from build123d import *

# Parameters (mm, degrees)
SKETCH1_R           = 22.5
BOSS_EXTRUDE1_DEPTH = 200
BOSS_EXTRUDE2_START = 50
BOSS_EXTRUDE2_DEPTH = 100
BOSS_EXTRUDE3_START = -50
SKETCH4_R           = 23.75
SKETCH4_R_2         = 22.25
BOSS_EXTRUDE3_DEPTH = 5
BOSS_EXTRUDE4_START = -171.5
SKETCH4_2_R         = 23.75
SKETCH4_2_R_2       = 22.25
BOSS_EXTRUDE4_DEPTH = 21.5


with BuildPart() as part:
    # Sketch1 → Boss-Extrude1 (new body)
    with BuildSketch(Plane.XY):
        Circle(SKETCH1_R)
        with BuildLine():
            Line((-3.5, 19.691368668), (-3.5, 17.656443583))
            ThreePointArc((-3.5, 17.656443583), (-6.888301783, 16.629831585), (-10.010117255, 14.959864723))
            Line((-10.010117255, 14.959864723), (-11.449026581, 16.39877405))
            ThreePointArc((-11.449026581, 16.39877405), (-14.142135624, 14.142135624), (-16.39877405, 11.449026581))
            Line((-16.39877405, 11.449026581), (-14.959864723, 10.010117255))
            ThreePointArc((-14.959864723, 10.010117255), (-16.629831585, 6.888301783), (-17.656443583, 3.5))
            Line((-17.656443583, 3.5), (-19.691368668, 3.5))
            ThreePointArc((-19.691368668, 3.5), (-20, 0), (-19.691368668, -3.5))
            Line((-19.691368668, -3.5), (-17.656443583, -3.5))
            ThreePointArc((-17.656443583, -3.5), (-16.629831585, -6.888301783), (-14.959864723, -10.010117255))
            Line((-14.959864723, -10.010117255), (-16.39877405, -11.449026581))
            ThreePointArc((-16.39877405, -11.449026581), (-14.142135624, -14.142135624), (-11.449026581, -16.39877405))
            Line((-11.449026581, -16.39877405), (-10.010117255, -14.959864723))
            ThreePointArc((-10.010117255, -14.959864723), (-6.888301783, -16.629831585), (-3.5, -17.656443583))
            Line((-3.5, -17.656443583), (-3.5, -19.691368668))
            ThreePointArc((-3.5, -19.691368668), (0, -20), (3.5, -19.691368668))
            Line((3.5, -19.691368668), (3.5, -17.656443583))
            ThreePointArc((3.5, -17.656443583), (6.888301783, -16.629831585), (10.010117255, -14.959864723))
            Line((10.010117255, -14.959864723), (11.449026581, -16.39877405))
            ThreePointArc((11.449026581, -16.39877405), (14.142135624, -14.142135624), (16.39877405, -11.449026581))
            Line((16.39877405, -11.449026581), (14.959864723, -10.010117255))
            ThreePointArc((14.959864723, -10.010117255), (16.629831585, -6.888301783), (17.656443583, -3.5))
            Line((17.656443583, -3.5), (19.691368668, -3.5))
            ThreePointArc((19.691368668, -3.5), (20, 0), (19.691368668, 3.5))
            Line((19.691368668, 3.5), (17.656443583, 3.5))
            ThreePointArc((17.656443583, 3.5), (16.629831585, 6.888301783), (14.959864723, 10.010117255))
            Line((14.959864723, 10.010117255), (16.39877405, 11.449026581))
            ThreePointArc((16.39877405, 11.449026581), (14.142135624, 14.142135624), (11.449026581, 16.39877405))
            Line((11.449026581, 16.39877405), (10.010117255, 14.959864723))
            ThreePointArc((10.010117255, 14.959864723), (6.888301783, 16.629831585), (3.5, 17.656443583))
            Line((3.5, 17.656443583), (3.5, 19.691368668))
            ThreePointArc((3.5, 19.691368668), (0, 20), (-3.5, 19.691368668))
        make_face(mode=Mode.SUBTRACT)
    extrude(amount=BOSS_EXTRUDE1_DEPTH)

    # Sketch3 → Boss-Extrude2 (add)
    with BuildSketch(Plane.XY.offset(BOSS_EXTRUDE2_START)):
        with BuildLine():
            Line((-2.000027302, 23.665962711), (-0.80077241, 26.237773126))
            ThreePointArc((-0.80077241, 26.237773126), (0, 26.249990002), (0.80077241, 26.237773126))
            Line((0.80077241, 26.237773126), (2.000027302, 23.665962711))
            ThreePointArc((2.000027302, 23.665962711), (2.731879206, 23.592683956), (3.461111111, 23.496778718))
            Line((3.461111111, 23.496778718), (3.461111111, 21.979153985))
            ThreePointArc((3.461111111, 21.979153985), (0, 22.25), (-3.461111111, 21.979153985))
            Line((-3.461111111, 21.979153985), (-3.461111111, 23.496778718))
            ThreePointArc((-3.461111111, 23.496778718), (-2.731879206, 23.592683956), (-2.000027302, 23.665962711))
        make_face()
        with BuildLine():
            Line((17.303950149, 13.98698714), (18.618251721, 14.745799506))
            ThreePointArc((18.618251721, 14.745799506), (19.065924046, 14.162218771), (19.495311261, 13.565055807))
            Line((19.495311261, 13.565055807), (22.322191861, 13.812375813))
            ThreePointArc((22.322191861, 13.812375813), (22.73315819, 13.124995001), (23.122964271, 12.425397313))
            Line((23.122964271, 12.425397313), (21.495338563, 10.100906903))
            ThreePointArc((21.495338563, 10.100906903), (21.797803252, 9.430465185), (22.079362832, 8.750979211))
            Line((22.079362832, 8.750979211), (20.76506126, 7.992166845))
            ThreePointArc((20.76506126, 7.992166845), (19.269065234, 11.125), (17.303950149, 13.98698714))
        make_face()
        with BuildLine():
            Line((20.76506126, -7.992166845), (22.079362832, -8.750979211))
            ThreePointArc((22.079362832, -8.750979211), (21.797803252, -9.430465185), (21.495338563, -10.100906903))
            Line((21.495338563, -10.100906903), (23.122964271, -12.425397313))
            ThreePointArc((23.122964271, -12.425397313), (22.73315819, -13.124995001), (22.322191861, -13.812375813))
            Line((22.322191861, -13.812375813), (19.495311261, -13.565055807))
            ThreePointArc((19.495311261, -13.565055807), (19.065924046, -14.162218771), (18.618251721, -14.745799506))
            Line((18.618251721, -14.745799506), (17.303950149, -13.98698714))
            ThreePointArc((17.303950149, -13.98698714), (19.269065234, -11.125), (20.76506126, -7.992166845))
        make_face()
        with BuildLine():
            Line((3.461111111, -21.979153985), (3.461111111, -23.496778718))
            ThreePointArc((3.461111111, -23.496778718), (2.731879206, -23.592683956), (2.000027302, -23.665962711))
            Line((2.000027302, -23.665962711), (0.80077241, -26.237773126))
            ThreePointArc((0.80077241, -26.237773126), (0, -26.249990002), (-0.80077241, -26.237773126))
            Line((-0.80077241, -26.237773126), (-2.000027302, -23.665962711))
            ThreePointArc((-2.000027302, -23.665962711), (-2.731879206, -23.592683956), (-3.461111111, -23.496778718))
            Line((-3.461111111, -23.496778718), (-3.461111111, -21.979153985))
            ThreePointArc((-3.461111111, -21.979153985), (0, -22.25), (3.461111111, -21.979153985))
        make_face()
        with BuildLine():
            Line((-17.303950149, -13.98698714), (-18.618251721, -14.745799506))
            ThreePointArc((-18.618251721, -14.745799506), (-19.065924046, -14.162218771), (-19.495311261, -13.565055807))
            Line((-19.495311261, -13.565055807), (-22.322191861, -13.812375813))
            ThreePointArc((-22.322191861, -13.812375813), (-22.73315819, -13.124995001), (-23.122964271, -12.425397313))
            Line((-23.122964271, -12.425397313), (-21.495338563, -10.100906903))
            ThreePointArc((-21.495338563, -10.100906903), (-21.797803252, -9.430465185), (-22.079362832, -8.750979211))
            Line((-22.079362832, -8.750979211), (-20.76506126, -7.992166845))
            ThreePointArc((-20.76506126, -7.992166845), (-19.269065234, -11.125), (-17.303950149, -13.98698714))
        make_face()
        with BuildLine():
            Line((-20.76506126, 7.992166845), (-22.079362832, 8.750979211))
            ThreePointArc((-22.079362832, 8.750979211), (-21.797803252, 9.430465185), (-21.495338563, 10.100906903))
            Line((-21.495338563, 10.100906903), (-23.122964271, 12.425397313))
            ThreePointArc((-23.122964271, 12.425397313), (-22.73315819, 13.124995001), (-22.322191861, 13.812375813))
            Line((-22.322191861, 13.812375813), (-19.495311261, 13.565055807))
            ThreePointArc((-19.495311261, 13.565055807), (-19.065924046, 14.162218771), (-18.618251721, 14.745799506))
            Line((-18.618251721, 14.745799506), (-17.303950149, 13.98698714))
            ThreePointArc((-17.303950149, 13.98698714), (-19.269065234, 11.125), (-20.76506126, 7.992166845))
        make_face()
    extrude(amount=BOSS_EXTRUDE2_DEPTH)

    # Sketch4 → Boss-Extrude3 (add)
    with BuildSketch(Plane.XY.offset(200).offset(BOSS_EXTRUDE3_START)):
        with Locations(Location((0, 0, 0), (0, 0, 180))):
            Circle(SKETCH4_R)
        Circle(SKETCH4_R_2, mode=Mode.SUBTRACT)
    extrude(amount=BOSS_EXTRUDE3_DEPTH)

    # Sketch4<2> → Boss-Extrude4 (add)
    with BuildSketch(Plane.XY.offset(200).offset(BOSS_EXTRUDE4_START)):
        with Locations(Location((0, 0, 0), (0, 0, 180))):
            Circle(SKETCH4_2_R)
        Circle(SKETCH4_2_R_2, mode=Mode.SUBTRACT)
    extrude(amount=BOSS_EXTRUDE4_DEPTH)


solid = part.part
Can you work these out from the model? Positions are in its coordinate system, mm. A direction names the side the tool comes from. Give positions to 0.01 mm unless a question says otherwise; leave off trailing zeros. Loops run counter-clockwise (first coordinate to the right, second up) from the corner with the lowest first, then second, coordinate; pieces in that order, holes last. Notation, with made-up numbers: M -2,51 L 49,51 A23 ccw 49,88 Z; hole C -37.75,-26 d6. An arc over 180 degrees is marked long. One line per item, written item: value.
1) Please list where these lines run through material, in increasing order: line 1 (X direction, y = -0.5, z = 106); line 2 (X direction, y = 16, z = 80); line 3 (X direction, y = 15.5, z = 149).
Geometry check:
line 1: x = -22.49 to -19.99, 19.99 to 22.49
line 2: x = -15.82 to -12, -11.05 to -8.25, 8.25 to 11.05, 12 to 15.82
line 3: x = -16.31 to -12.64, -10.55 to -9.15, 9.15 to 10.55, 12.64 to 16.31
2) Imagine slicing it at A-A on y = 0. Write out the boundary of the cut face in (x, z), and give its area (3 significant figures).
Geometry check:
outline: M -23.75,28.5 L -22.5,28.5 L -22.5,0 L -20,0 L -20,200 L -22.5,200 L -22.5,155 L -23.75,155 L -23.75,150 L -22.5,150 L -22.5,50 L -23.75,50 Z; M 20,0 L 22.5,0 L 22.5,28.5 L 23.75,28.5 L 23.75,50 L 22.5,50 L 22.5,150 L 23.75,150 L 23.75,155 L 22.5,155 L 22.5,200 L 20,200 Z
area: 1,070 mm²
3) Thinking about a two-plate mould opening in Y: for faces 5 (the face through (-21, 12, 150)), 6 (the face through (-11.149, 19.543, 99.3)), 7 (the face through (20, 0, 99)), which applies, +Y half, -Y half, draft (parallel to the pull), parting line (faces both ways), or undercut?
Geometry check:
face 5: draft
face 6: +Y half
face 7: undercut
4) I'm going to push flat-ended pins straight in: pin 1 (0.6 mm diameter, centred on y = -23, z = 107, fed in from -X); pin 2 (1.4 mm diameter, centred on x = 1, y = -24.5, fed in from +Z); pin 3 (12 mm diameter, centred on x = -16.5, z = 29, fed in from -Y); pin 4 (3 mm diameter, centred on x = 22, y = 0.5, fed in from -Z). Where does each tip first touch, or does it pass through?
Geometry check:
pin 1: stops at x = -3.46
pin 2: stops at z = 150
pin 3: stops at y = -21.3
pin 4: stops at z = 0
5) On a 3-axis mill with a long thin cutter (end or side, diameter ignored), from which of +Z, -Z, +X, -X, +Y, -Y can I reach the whole of each face in a straight line? I mean faces 1 (the face through (0, 20, 99)), 2 (the face through (-21, 12, 50)), 3 (the face through (22, 12, 150)), 4 (the face through (-21, 9, 155)). Say none if no direction works.
Geometry check:
face 1: +Z, -Z
face 2: -Z, -X, +Y
face 3: +Z, +X, +Y
face 4: +Z
6) Imagine slicing it at C-C on x = 7.5. Write out the boundary of the cut face in (y, z).
Geometry check:
outline: M -22.53,28.5 L -21.21,28.5 L -21.21,0 L -16.36,0 L -16.36,200 L -21.21,200 L -21.21,155 L -22.53,155 L -22.53,150 L -21.21,150 L -21.21,50 L -22.53,50 Z; M 16.36,0 L 21.21,0 L 21.21,28.5 L 22.53,28.5 L 22.53,50 L 21.21,50 L 21.21,150 L 22.53,150 L 22.53,155 L 21.21,155 L 21.21,200 L 16.36,200 Z
